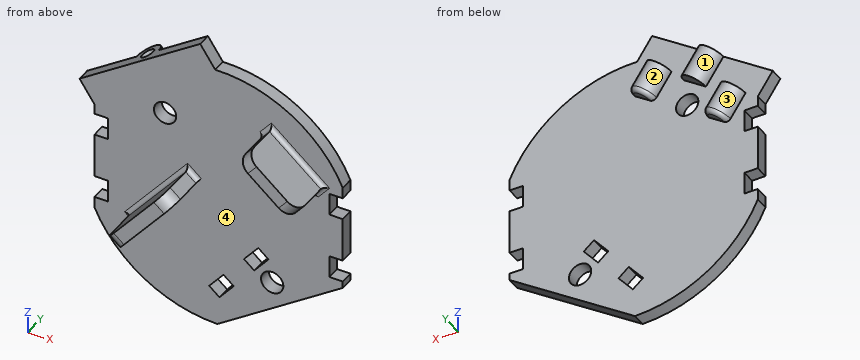
from build123d import *

# Parameters (mm, degrees)
CROQUIS1_R              = 30.5
SALIENTE_EXTRUIR1_DEPTH = 3
CORTAR_EXTRUIR3_START   = -4
CORTAR_EXTRUIR3_DEPTH   = 4
CORTAR_EXTRUIR6_DEPTH   = 10
CROQUIS10_R             = 2.5
CORTAR_EXTRUIR7_DEPTH   = 10
CORTAR_EXTRUIR8_START   = -3
CORTAR_EXTRUIR8_DEPTH   = 3
SALIENTE_EXTRUIR2_DEPTH = 10
REDONDEO1_R             = 3
REDONDEO2_R             = 1
CORTAR_EXTRUIR9_START   = -3
CORTAR_EXTRUIR9_DEPTH   = 3
CORTAR_EXTRUIR10_START  = -10
CORTAR_EXTRUIR10_DEPTH  = 10
CROQUIS19_R             = 3
SALIENTE_EXTRUIR5_DEPTH = 7
CROQUIS20_R             = 1.5
CORTAR_EXTRUIR12_DEPTH  = 6
REDONDEO3_R             = 1
CROQUIS16_W             = 32.622025527
CROQUIS16_H             = 3
SALIENTE_EXTRUIR3_DEPTH = 6
CROQUIS17_R             = 3
SALIENTE_EXTRUIR4_DEPTH = 7
CROQUIS18_R             = 1.5
CORTAR_EXTRUIR11_DEPTH  = 6


with BuildPart() as part:
    # Croquis1 → Saliente-Extruir1 (new body)
    with BuildSketch(Plane(origin=(0, 0, 0), x_dir=(1, 0, 0), z_dir=(0, 1, 0))):
        with Locations(Location((0, 0, 0), (0, 0, 270))):
            Circle(CROQUIS1_R)
    extrude(amount=SALIENTE_EXTRUIR1_DEPTH)

    # Croquis5 → Cortar-Extruir3 (cut)
    with BuildSketch(Plane(origin=(0, 3, 0), x_dir=(1, 0, 0), z_dir=(0, 1, 0)).offset(CORTAR_EXTRUIR3_START)):
        with BuildLine():
            Line((28.814059068, 5), (30.087372767, 5))
            ThreePointArc((30.087372767, 5), (29.556634924, 7.526973624), (28.814059068, 10))
            Line((28.814059068, 10), (24.814059068, 10))
            Line((24.814059068, 10), (24.814059068, 5))
            Line((24.814059068, 5), (28.814059068, 5))
        make_face()
        with BuildLine():
            Line((30.087372767, -5), (28.814059068, -5))
            Line((28.814059068, -5), (24.814059068, -5))
            Line((24.814059068, -5), (24.814059068, -10))
            Line((24.814059068, -10), (28.814059068, -10))
            ThreePointArc((28.814059068, -10), (29.556634924, -7.526973624), (30.087372767, -5))
        make_face()
        with BuildLine():
            Line((-24.814059068, 5), (-24.814059068, 10))
            Line((-24.814059068, 10), (-28.814059068, 10))
            ThreePointArc((-28.814059068, 10), (-29.556634924, 7.526973624), (-30.087372767, 5))
            Line((-30.087372767, 5), (-28.814059068, 5))
            Line((-28.814059068, 5), (-24.814059068, 5))
        make_face()
        with BuildLine():
            Line((-28.814059068, -10), (-24.814059068, -10))
            Line((-24.814059068, -10), (-24.814059068, -5))
            Line((-24.814059068, -5), (-28.814059068, -5))
            Line((-28.814059068, -5), (-30.087372767, -5))
            ThreePointArc((-30.087372767, -5), (-29.556634924, -7.526973624), (-28.814059068, -10))
        make_face()
    extrude(amount=CORTAR_EXTRUIR3_DEPTH, mode=Mode.SUBTRACT)

    # Croquis9 → Cortar-Extruir6 (cut)
    with BuildSketch(Plane(origin=(0, 3, 0), x_dir=(1, 0, 0), z_dir=(0, 1, 0))):
        Polygon((5.673284852, 12.685390231), (8.887222901, 8.855168016), (11.18535623, 10.783530845), (7.971418181, 14.613753061), align=None)
        Polygon((-2.120514915, 21.973679104), (1.093423133, 18.143456889), (3.391556462, 20.071819718), (0.177618414, 23.902041933), align=None)
    extrude(amount=-CORTAR_EXTRUIR6_DEPTH, mode=Mode.SUBTRACT)

    # Croquis10 → Cortar-Extruir7 (cut)
    with BuildSketch(Plane(origin=(0, 3, 0), x_dir=(1, 0, 0), z_dir=(0, 1, 0))):
        with Locations(Location((12, 16, 0), (0, 0, 270))):
            Circle(CROQUIS10_R)
        with Locations(Location((-12, -16, 0), (0, 0, 270))):
            Circle(CROQUIS10_R)
    extrude(amount=-CORTAR_EXTRUIR7_DEPTH, mode=Mode.SUBTRACT)

    # Croquis11 → Cortar-Extruir8 (cut)
    with BuildSketch(Plane(origin=(0, 3, 0), x_dir=(1, 0, 0), z_dir=(0, 1, 0)).offset(CORTAR_EXTRUIR8_START)):
        with BuildLine():
            ThreePointArc((-28.814059068, -10), (-28.341972277, -11.268655974), (-27.814059068, -12.515115586))
            Line((-27.814059068, -12.515115586), (-27.814059068, -10))
            Line((-27.814059068, -10), (-28.814059068, -10))
        make_face()
        with BuildLine():
            Line((-27.814059068, -5), (-27.814059068, 5))
            Line((-27.814059068, 5), (-30.087372767, 5))
            ThreePointArc((-30.087372767, 5), (-30.5, 0), (-30.087372767, -5))
            Line((-30.087372767, -5), (-27.814059068, -5))
        make_face()
        with BuildLine():
            Line((-27.814059068, 10), (-27.814059068, 12.515115586))
            ThreePointArc((-27.814059068, 12.515115586), (-28.341972277, 11.268655974), (-28.814059068, 10))
            Line((-28.814059068, 10), (-27.814059068, 10))
        make_face()
        with BuildLine():
            Line((28.814059068, -10), (27.814059068, -10))
            Line((27.814059068, -10), (27.814059068, -12.515115586))
            ThreePointArc((27.814059068, -12.515115586), (28.341972277, -11.268655974), (28.814059068, -10))
        make_face()
        with BuildLine():
            Line((30.087372767, 5), (27.814059068, 5))
            Line((27.814059068, 5), (27.814059068, -5))
            Line((27.814059068, -5), (30.087372767, -5))
            ThreePointArc((30.087372767, -5), (30.5, 0), (30.087372767, 5))
        make_face()
        with BuildLine():
            Line((27.814059068, 12.515115586), (27.814059068, 10))
            Line((27.814059068, 10), (28.814059068, 10))
            ThreePointArc((28.814059068, 10), (28.341972277, 11.268655974), (27.814059068, 12.515115586))
        make_face()
    extrude(amount=CORTAR_EXTRUIR8_DEPTH, mode=Mode.SUBTRACT)

    # Croquis13 → Saliente-Extruir2 (add)
    with BuildSketch(Plane.XZ):
        Polygon((-6.816688183, 4.321977983), (-19.672440377, -10.99891088), (-17.374307048, -12.927273709), (-4.518554854, 2.393615154), align=None)
        Polygon((21.527275636, 8.931176939), (23.455638465, 11.229310268), (11.964971818, 20.871124414), (10.036608989, 18.572991084), align=None)
    extrude(amount=SALIENTE_EXTRUIR2_DEPTH)

    # Redondeo1
    redondeo1_edges = [part.edges().sort_by_distance(p)[0] for p in [
        (-5.667621519, -10, 3.357796568),
        (-18.523373712, -10, -11.963092294),
        (22.49145705, -10, 10.080243604),
        (11.000790403, -10, 19.722057749),
    ]]
    fillet(redondeo1_edges, radius=REDONDEO1_R)

    # Redondeo2
    redondeo2_edges = [part.edges().sort_by_distance(p)[0] for p in [
        (-5.667621519, 0, 3.357796568),
        (-13.24456428, 0, -3.338466449),
        (-18.523373712, 0, -11.963092294),
        (22.49145705, 0, 10.080243604),
        (17.710305141, 0, 16.050217341),
        (11.000790403, 0, 19.722057749),
    ]]
    fillet(redondeo2_edges, radius=REDONDEO2_R)

    # Croquis14 → Cortar-Extruir9 (cut)
    with BuildSketch(Plane(origin=(0, 3, 0), x_dir=(1, 0, 0), z_dir=(0, 1, 0)).offset(CORTAR_EXTRUIR9_START)):
        with BuildLine():
            Line((-0.28585192, 30.498660441), (27.814059068, 11.545031156))
            Line((27.814059068, 11.545031156), (27.814059068, 12.515115586))
            ThreePointArc((27.814059068, 12.515115586), (16.440879495, 25.689442995), (-0.28585192, 30.498660441))
        make_face()
    extrude(amount=CORTAR_EXTRUIR9_DEPTH, mode=Mode.SUBTRACT)

    # Croquis15 → Cortar-Extruir10 (cut)
    with BuildSketch(Plane(origin=(0, 3, 0), x_dir=(1, 0, 0), z_dir=(0, 1, 0)).offset(CORTAR_EXTRUIR10_START)):
        with BuildLine():
            Line((-27.814059068, -12.24829445), (-27.814059068, -12.515115586))
            ThreePointArc((-27.814059068, -12.515115586), (-16.882746118, -25.401237834), (-0.769174213, -30.490299622))
            Line((-0.769174213, -30.490299622), (-27.814059068, -12.24829445))
        make_face()
    extrude(amount=CORTAR_EXTRUIR10_DEPTH, mode=Mode.SUBTRACT)

    # Croquis19 → Saliente-Extruir5 (add)
    with BuildSketch(Plane(origin=(-14.375575006, 0, 21.312666404), x_dir=(0.8290375725550415, 0, 0.5591929034707471), z_dir=(-0.5591929034707471, 0, 0.8290375725550415))):
        with Locations((10.101272087, 3)):
            Circle(CROQUIS19_R)
        with Locations((-9.898727913, 3)):
            Circle(CROQUIS19_R)
    extrude(amount=-SALIENTE_EXTRUIR5_DEPTH)

    # Croquis20 → Cortar-Extruir12 (cut)
    with BuildSketch(Plane(origin=(-14.375575006, 0, 21.312666404), x_dir=(0.8290375725550415, 0, 0.5591929034707471), z_dir=(-0.5591929034707471, 0, 0.8290375725550415))):
        with Locations((10.101272087, 3)):
            Circle(CROQUIS20_R)
        with Locations((-9.898727913, 3)):
            Circle(CROQUIS20_R)
    extrude(amount=-CORTAR_EXTRUIR12_DEPTH, mode=Mode.SUBTRACT)

    # Redondeo3
    redondeo3_edges = [part.edges().sort_by_distance(p)[0] for p in [
        (-2.086890591, 6, 21.157963063),
        (-18.667642042, 6, 9.974104993),
    ]]
    fillet(redondeo3_edges, radius=REDONDEO3_R)

    # Croquis16 → Saliente-Extruir3 (add)
    with BuildSketch(Plane(origin=(-14.375575006, 0, 21.312666404), x_dir=(0.8290375725550415, 0, 0.5591929034707471), z_dir=(-0.5591929034707471, 0, 0.8290375725550415))):
        with Locations((0.101272086, 1.5)):
            Rectangle(CROQUIS16_W, CROQUIS16_H)
    extrude(amount=SALIENTE_EXTRUIR3_DEPTH)

    # Croquis17 → Saliente-Extruir4 (add)
    with BuildSketch(Plane(origin=(-17.730732427, 0, 26.286891839), x_dir=(0.8290375725550415, 0, 0.5591929034707471), z_dir=(-0.5591929034707471, 0, 0.8290375725550415))):
        with Locations((0.101272087, 3)):
            Circle(CROQUIS17_R)
    extrude(amount=-SALIENTE_EXTRUIR4_DEPTH)

    # Croquis18 → Cortar-Extruir11 (cut)
    with BuildSketch(Plane(origin=(-17.730732427, 0, 26.286891839), x_dir=(0.8290375725550415, 0, 0.5591929034707471), z_dir=(-0.5591929034707471, 0, 0.8290375725550415))):
        with Locations((0.101272087, 3)):
            Circle(CROQUIS18_R)
    extrude(amount=-CORTAR_EXTRUIR11_DEPTH, mode=Mode.SUBTRACT)


solid = part.part
Design review of the part built by this model. Coordinates are the model's own, in mm. Face numbers are marked on the shaded views. Give positions to 0.01 mm unless a question says otherwise; leave off trailing zeros. Loops run counter-clockwise (first coordinate to the right, second up) from the corner with the lowest first, then second, coordinate; pieces in that order, holes last. Notation, with made-up numbers: M 35.25,-10.5 L 61.25,-10.5 A22 ccw 61.25,6.5 Z; hole C -38,3 d11. An arc over 180 degrees is marked long. Write item = value, one per line.
Q1. To check wall thickness, follow line 1 (X direction, y = 3.75, z = 26); line 2 (X direction, y = 2.25, z = 16); line 3 (Z direction, x = 1.5, y = 2.25). State the ranges of each line that lie inside material, in increasing order. Write a range as [from, to].
Output values:
line_1 = [-15.85, -13.91], [-7.43, -6.92], [-3.79, -1.85]
line_2 = [-30.34, -22.25], [-21.17, -14.5], [-9.5, 25.97]
line_3 = [-29.29, -22.33], [-18.48, 30.46]
Q2. Insertion check: pin 1 (1.5 mm diameter, centred on y = 3.5, z = 7, fed in from +X); pin 2 (1.5 mm diameter, centred on y = 2, z = 21.5, fed in from -X); pin 3 (5 mm diameter, centred on y = 0, z = -1.5, fed in from -X); pin 4 (1 mm diameter, centred on y = -5, z = -14, fed in from -X). Each pin has a flat end and moves straight along its axis. Give the tip position at first contact, or say it passes through.
Output values:
pin_1 = 24.81
pin_2 = -25.94
pin_3 = -27.81
pin_4 = through
Q3. Draft analysis for pull direction X (two halves, no side actions). For the marked faces 1, 2, 3 and 4, state which applies: +X half, -X half, draft (parallel to the pull), parting line (faces both ways), or undercut.
Output values:
face_1 = undercut
face_2 = undercut
face_3 = parting line
face_4 = draft
Q4. We need section D-D (z = -25.5). Give the boundary of the cut face in (x, y), plus the area to 3 significant figures.
Output values:
outline = M -16.73,0 L 7.12,0 L 7.12,3 L -16.73,3 Z
area = 71.6 mm^2
Q5. We need section A-A (y = -4.5). Give the boundary of the cut face in (x, z), plus the area to 3 significant figures.
Output values:
outline = M -19.67,-11 L -17.37,-12.93 L -4.52,2.39 L -6.82,4.32 Z; M 10.04,18.57 L 21.53,8.93 L 23.46,11.23 L 11.96,20.87 Z
area = 105 mm^2
Q6. We need section B-B (z = -16). Give the boundary of the cut face in (x, y), plus the area to 3 significant figures.
Output values:
outline = M -25.97,0 L 9.5,0 L 9.5,3 L -25.97,3 Z; M 14.5,0 L 21.21,0 L 21.21,3 L 14.5,3 Z
area = 127 mm^2
Q7. We need section C-C (x = -26). Give the boundary of the cut face in (y, z), plus the area to 3 significant figures.
Output values:
outline = M 0,-15.95 L 3,-15.95 L 3,-10 L 0,-10 Z; M 0,-5 L 3,-5 L 3,5 L 0,5 Z; M 0,10 L 3,10 L 3,20.71 L 0,20.71 Z
area = 80.0 mm^2
